Autodesk Inventor part; units mm, degrees
ref_plane "YZ Plane" through (0, 0, 0) normal (1, 0, 0) x (0, 1, 0)
ref_plane "XZ Plane" through (0, 0, 0) normal (0, 1, 0) x (-1, 0, 0)
ref_plane "XY Plane" through (0, 0, 0) normal (0, 0, 1) x (1, 0, 0)
sketch "Sketch1" plane through (0, 0, 0) normal (0, 0, 1) x (1, 0, 0)
  line L0 (-27.5, 15) -> (27.5, 15)
  line L1 (27.5, 15) -> (27.5, -15)
  line L2 (27.5, -15) -> (-27.5, -15)
  line L3 (-27.5, -15) -> (-27.5, 15)
  point P0 (0, 0)
  point P1 (0, 15)
  point P2 (-27.5, 0)
  dimension "d0" = 55
  dimension "d1" = 30
extrude "Extrusion1" add sketch "Sketch1" along normal blind 8
sketch "Sketch5" plane through (0, 0, 8) normal (0, 0, 1) x (1, 0, 0)
  line L0 (12.5, 11) -> (-22.5, 11) construction
  line L1 (12.5, 12.75) -> (-22.5, 12.75)
  line L2 (-22.5, 9.25) -> (12.5, 9.25)
  arc A0 (12.5, 9.25) -> (12.5, 12.75) centre (12.5, 11) ccw
  arc A1 (-22.5, 12.75) -> (-22.5, 9.25) centre (-22.5, 11) ccw
  line L3 (12.5, -11) -> (-22.5, -11) construction
  line L4 (12.5, -9.25) -> (-22.5, -9.25)
  line L5 (-22.5, -12.75) -> (12.5, -12.75)
  arc A2 (12.5, -12.75) -> (12.5, -9.25) centre (12.5, -11) ccw
  arc A3 (-22.5, -9.25) -> (-22.5, -12.75) centre (-22.5, -11) ccw
  line L6 (27.5, 15) -> (-27.5, 15)
  line L7 (-27.5, -15) -> (27.5, -15)
  line L8 (-27.5, 15) -> (-27.5, -15)
  point P0 (0, 0)
  point P1 (-5, 11)
  point P2 (-5, -11)
  dimension "d29" = 3.5
  dimension "d30" = 4
  dimension "d31" = 4
  dimension "d33" = 35
  dimension "d36" = 5
extrude "Extrusion5" cut sketch "Sketch5" against normal blind 10
sketch "Sketch6" plane through (0, 0, 8) normal (0, 0, 1) x (1, 0, 0)
  circle A0 centre (24.3725, -11.7625) radius 1.7875
  circle A1 centre (24.3725, 7.4125) radius 1.7875
  line L0 (27.5, -15) -> (27.5, 15)
  point P0 (0, 0)
  dimension "d44" = 3.1275
hole "Hole1" at (24.3725, 7.4125, 8) at (24.3725, -11.7625, 8) direction (0, 0, -1) diameter 2.459 end through all
properties part number "0005-10-021 suport senzor z"
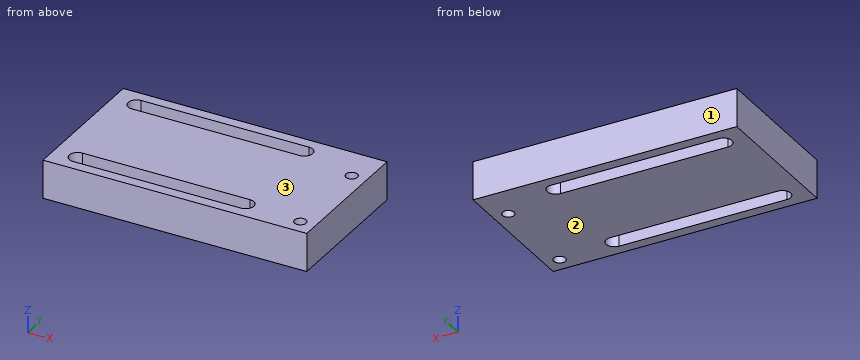
The listing builds one solid part. Answer for the finished solid, in the listing's coordinates (mm). Face numbers are marked on the shaded views. Give positions to 0.01 mm unless a question says otherwise; leave off trailing zeros. Loops run counter-clockwise (first coordinate to the right, second up) from the corner with the lowest first, then second, coordinate; pieces in that order, holes last. Notation, with made-up numbers: M 47.5,1.25 L 91.5,1.25 A27 cw 91.5,17.25 Z; hole C -7.5,65 d3. An arc over 180 degrees is marked long. One line per item, written item: value.
Q1. A cutting plane is placed at A-A on y = 11. Determine the outline of the cut face in (x, z), then the cut area to 3 significant figures.
Working result:
outline: M -27.5,0 L -24.25,0 L -24.25,8 L -27.5,8 Z; M 14.25,0 L 27.5,0 L 27.5,8 L 14.25,8 Z
area: 132 mm^2
Q2. A cutting plane is placed at C-C on y = 8. Determine the outline of the cut face in (x, z), then the cut area to 3 significant figures.
Working result:
outline: M -27.5,0 L 23.29,0 L 23.29,8 L -27.5,8 Z; M 25.45,0 L 27.5,0 L 27.5,8 L 25.45,8 Z
area: 423 mm^2
Q3. Find the intervals of material crossed by line 1 (Y direction, x = -1.5, z = 7.75); line 2 (X direction, y = 7.5, z = 0.5); line 3 (X direction, y = 12.25, z = 1.5), in increasing order. Write a range as from..to.
Working result:
line 1: y = -15..-12.75, -9.25..9.25, 12.75..15
line 2: x = -27.5..23.15, 25.6..27.5
line 3: x = -27.5..-23.72, 13.72..27.5
Q4. Determine the mould class of the marked faces 1, 2 and 3 for opening direction Z: +Z half, -Z half, draft (parallel to the pull), parting line (faces both ways), or undercut.
Working result:
face 1: draft
face 2: -Z half
face 3: +Z half
Q5. A cutting plane is placed at B-B on z = 5.25. Determine the outline of the cut face in (x, y).
Working result:
outline: M -27.5,-15 L 27.5,-15 L 27.5,15 L -27.5,15 Z; hole M -22.5,-12.75 L 12.5,-12.75 A1.75 ccw 12.5,-9.25 L -22.5,-9.25 A1.75 ccw Z; hole M -22.5,9.25 L 12.5,9.25 A1.75 ccw 12.5,12.75 L -22.5,12.75 A1.75 ccw Z; hole C 24.37,-11.76 d2.46; hole C 24.37,7.41 d2.46
